Build history of the part. All positions in model axes, mm. A direction names the side the tool comes from. Give positions to 0.01 mm unless a question says otherwise; leave off trailing zeros. Order: outer loops, then holes, each group sorted by start corner. A loop starts at its lowest first (then second) coordinate and runs counter-clockwise, first axis right, second up. Notation, with made-up numbers: (-11.75, 46) - (45.25, 46) arc R31 ccw to (45.25, 75) - close; hole circle Ø4 at (27, 68.25). An arc over 180 degrees is marked (long way). Use a Markdown table: item, result. Add a question column.
(1) Which spindle directions (+Z, -Z, +X, -X, +Y, -Y) get a long thin tool onto all of the face, cutting with end or side? Do faces 1 (the face through (-19, 78, 4)), 2 (the face through (-1, 21, 6)), 3 (the face through (0, 6, 3)). Say none if no direction does.
(2) Slice it at C-C (x = -13). Write the cut outline in (y, z).
(3) Slice it at A-A (y = 38). Write the cut outline in (x, z), then the cut area to 3 significant figures.
(4) Slice it at B-B (x = -1.5). Write the cut outline in (y, z), then the cut area to 3 significant figures.
(5) Flat gauge pins, fed straight in: pin 1 (1.5 mm diameter, centred on y = 57, z = 1, fed in from +X); pin 2 (1.5 mm diameter, centred on y = 104, z = 5.5, fed in from +X); pin 3 (7.5 mm diameter, centred on x = 9.5, y = 64, fed in from +Z). Where does each tip first touch, or does it go through?
(6) Wall check: line 1 (Y direction, x = 12, z = 6.5); line 2 (X direction, y = 12, z = 1); line 3 (Y direction, x = -1.5, z = 0.5). Give the ranges that are in metal, low to high.
Autodesk Inventor part; units mm, degrees
ref_plane "SunkenDetailsPlane" through (0, 0, 9) normal (0, 0, 1) x (1, 0, 0)
ref_plane "HolesPlane" through (-11, 95.6898, 6.5) normal (0, 0, 1) x (1, 0, 0)
ref_plane "YZ Plane" through (0, 0, 0) normal (1, 0, 0) x (0, 1, 0)
sketch "Base" plane through (0, 0, 0) normal (0, 0, 1) x (1, 0, 0)
  line L0 (0, -40.5971) -> (0, 168.3327) construction
  arc A0 (-10.75, 0) -> (10.75, 0) centre (0, 0) ccw
  line L1 (10.75, 48) -> (10.75, 0)
  line L2 (-10.75, 0) -> (-10.75, 50)
  line L3 (-19, 62.5716) -> (-16.2211, 52.5512)
  line L4 (-10.75, 50) -> (-16.2211, 52.5512)
  line L5 (-19, 62.5716) -> (-19, 93.5716)
  line L6 (-19, 93.5716) -> (-11.2142, 103.5369)
  line L7 (10.75, 48) -> (46.4584, 93.7046)
  line L8 (46.4584, 93.7046) -> (52.0821, 118.0639)
  arc A1 (52.0821, 118.0639) -> (48.6133, 127.8595) centre (42.6597, 120.2392) ccw
  arc A2 (48.6133, 127.8595) -> (35.0394, 126.1928) centre (42.6597, 120.2392) ccw
  line L9 (34.8364, 125.933) -> (20.2582, 137.3228)
  line L10 (35.0394, 126.1928) -> (34.8364, 125.933)
  arc A3 (20.2582, 137.3228) -> (14.6435, 136.6334) centre (17.7956, 134.1707) ccw
  line L11 (14.6435, 136.6334) -> (-11.2142, 103.5369)
  line L12 (42.6597, 120.2392) -> (48.6133, 127.8595) construction
  dimension "d0" = 142
  dimension "d1" = 155
  dimension "d2" = 21.5
  dimension "d3" = 115
  dimension "d4" = 130.5
  dimension "d7" = 51.5
  dimension "d8" = 18.5
  dimension "d9" = 4
  dimension "d10" = 58
  dimension "d11" = 25
  dimension "d14" = 42
  dimension "d15" = 50
  dimension "d18" = 10
  dimension "d57" = 48
  dimension "d100" = 19
  dimension "d101" = 31
extrude "BaseFeature" add sketch "Base" along normal blind 9
ref_plane "SunkenDetailsPlane" through (0, 0, 9) normal (0, 0, 1) x (1, 0, 0)
sketch "SunkenDetails" plane through (0, 0, 9) normal (0, 0, 1) x (1, 0, 0)
  line L0 (0.9151, 89.8249) -> (26.6729, 122.7934)
  line L1 (4.8551, 86.7466) -> (30.613, 119.7151)
  arc A0 (30.613, 119.7151) -> (26.6729, 122.7934) centre (28.6429, 121.2543) ccw
  line L2 (0.9151, 97.9462) -> (24.272, 127.8418)
  line L3 (24.272, 127.8418) -> (20.332, 130.9201)
  line L4 (16.1209, 130.403) -> (0.9151, 110.9404)
  arc A1 (20.332, 130.9201) -> (16.1209, 130.403) centre (18.485, 128.556) ccw
  line L5 (-4, 91.6552) -> (-4, 104.6494)
  line L6 (-4, 104.6494) -> (-11, 95.6898)
  line L7 (-11, 95.6898) -> (-11, 55.6335)
  line L8 (-11, 55.6335) -> (-4, 52.3693)
  line L9 (-4, 77.8836) -> (-4, 52.3693)
  arc A2 (-6.1033, 88.9631) -> (-4, 77.8836) centre (-0.1932, 84.3457) ccw
  line L10 (-6.1033, 88.9631) -> (-4, 91.6552)
  line L11 (5.75, 42.3059) -> (5.75, 0)
  line L12 (-5.75, 47.6685) -> (5.75, 42.3059)
  line L13 (-5.75, 0) -> (-5.75, 47.6685)
  arc A3 (-5.75, 0) -> (5.75, 0) centre (0, 0) ccw
  line L14 (4.6626, 48.3299) -> (26.8264, 76.6983)
  line L15 (3.3496, 76.6983) -> (26.8264, 76.6983)
  line L16 (1, 73.6909) -> (3.3496, 76.6983)
  arc A4 (0.9151, 89.8249) -> (4.8551, 86.7466) centre (2.8851, 88.2857) ccw
  line L17 (7.256, 81.6983) -> (30.7329, 81.6983)
  line L18 (7.256, 81.6983) -> (39.1705, 122.5469)
  line L19 (30.7329, 81.6983) -> (41.8359, 95.9094)
  line L20 (41.8359, 95.9094) -> (47.1112, 118.7594)
  arc A5 (47.1112, 118.7594) -> (39.1705, 122.5469) centre (42.721, 119.7729) ccw
  line L21 (10.75, 0) -> (10.75, 48) construction
  arc A6 (-10.75, 0) -> (10.75, 0) centre (0, 0) ccw construction
  line L22 (10.75, 0) -> (10.75, 48) construction
  line L23 (10.75, 48) -> (46.4584, 93.7046) construction
  line L24 (46.4584, 93.7046) -> (52.0821, 118.0639) construction
  arc A7 (52.0821, 118.0639) -> (35.0394, 126.1928) centre (42.6597, 120.2392) ccw construction
  line L25 (35.0394, 126.1928) -> (34.8364, 125.933) construction
  line L26 (34.8364, 125.933) -> (20.2582, 137.3228) construction
  arc A8 (20.2582, 137.3228) -> (14.6435, 136.6334) centre (17.7956, 134.1707) ccw construction
  line L27 (14.6435, 136.6334) -> (-19, 93.5716) construction
  line L28 (-19, 93.5716) -> (-19, 62.5716) construction
  line L29 (-19, 62.5716) -> (-16.2211, 52.5512) construction
  line L30 (-16.2211, 52.5512) -> (-10.75, 50) construction
  line L31 (-10.75, 50) -> (-10.75, 0) construction
  line L32 (-10.75, 50) -> (-10.75, 0) construction
  line L33 (10.75, 48) -> (46.4584, 93.7046) construction
  line L34 (-19, 93.5716) -> (-19, 62.5716) construction
  line L35 (14.6435, 136.6334) -> (-19, 93.5716) construction
  line L36 (46.4584, 93.7046) -> (52.0821, 118.0639) construction
  line L37 (34.8364, 125.933) -> (20.2582, 137.3228) construction
  arc A9 (-10.75, 0) -> (10.75, 0) centre (0, 0) ccw construction
  line L38 (24.272, 127.8418) -> (30.1821, 123.2243) construction
  line L39 (-10.75, 50) -> (-5.75, 47.6685) construction
  line L40 (-16.2211, 52.5512) -> (-10.75, 50) construction
  line L41 (2.8851, 88.2857) -> (-0.1932, 84.3457) construction
  line L42 (0.9151, 110.9404) -> (0.9151, 97.9462)
  line L43 (0.9151, 97.9462) -> (-4, 91.6552) construction
  line L44 (0.9151, 97.9462) -> (0.9151, 89.8249) construction
  line L45 (39.1705, 122.5469) -> (34.8364, 125.933) construction
  line L46 (1.346, 86.3157) -> (7.256, 81.6983) construction
  line L47 (1, 73.6909) -> (1, 50.0378)
  line L48 (1, 50.0378) -> (4.6626, 48.3299)
  point P0 (-11.2142, 103.5369)
  dimension "d23" = 5
  dimension "d30" = 8
  dimension "d32" = 5
  dimension "d34" = 5
  dimension "d35" = 5
  dimension "d36" = 5
  dimension "d49" = 5
  dimension "d54" = 5
  dimension "d59" = 5
  dimension "d60" = 5
  dimension "d61" = 5
  dimension "d66" = 5
  dimension "d76" = 3
  dimension "d77" = 7
  dimension "d102" = 5
  dimension "d103" = 5
  dimension "d104" = 36
extrude "SunkenDetailsFeature" cut sketch "SunkenDetails" against normal blind 5 contours L0 A0 L1 A4 | L42 L4 A1 L3 L2 | L10 A2 L9 L8 L7 L6 L5 | L48 L47 L16 L15 L14 | L18 A5 L20 L19 L17
ref_plane "HolesPlane" through (-11, 95.6898, 6.5) normal (0, 0, 1) x (1, 0, 0)
sketch "Holes" plane through (-11, 95.6898, 6.5) normal (0, 0, 1) x (1, 0, 0)
  circle A0 centre (21.6537, 21.2184) radius 3
  circle A1 centre (28.426, 29.8865) radius 3
  circle A2 centre (11, -57.6898) radius 3
  circle A3 centre (11, -68.6898) radius 3
  line L0 (8, -77.6898) -> (8, -86.6898)
  arc A4 (8, -86.6898) -> (14, -86.6898) centre (11, -86.6898) ccw
  line L1 (14, -86.6898) -> (14, -77.6898)
  arc A5 (14, -77.6898) -> (8, -77.6898) centre (11, -77.6898) ccw
  circle A6 centre (11, -95.6898) radius 3
  line L2 (11.9151, 15.2506) -> (27.1209, 34.7132) construction
  line L3 (35.272, 32.152) -> (11.9151, 2.2564) construction
  line L4 (21.6537, 21.2184) -> (28.426, 29.8865) construction
  line L5 (31.332, 35.2303) -> (35.272, 32.152)
  arc A7 (0.25, -95.6898) -> (21.75, -95.6898) centre (11, -95.6898) ccw construction
  line L6 (0.25, -45.6898) -> (0.25, -95.6898) construction
  line L7 (21.75, -95.6898) -> (21.75, -47.6898) construction
  line L8 (11, -57.6898) -> (11, -95.6898) construction
  dimension "d83" = 6
  dimension "d84" = 9
  dimension "d85" = 9
  dimension "d86" = 9
  dimension "d87" = 11
  dimension "d88" = 8
  dimension "d89" = 11
  dimension "d90" = 4
  dimension "d91" = 6
extrude "HolesFeature" cut sketch "Holes" against normal through all
extrude "SunkenDetailFeature" cut sketch "SunkenDetails" against normal blind 3 contours L11 A3 L13 L12
chamfer "DetailChamfersFeature" distance 1 angle 45 9 edges at (0.9151, 97.9462, 6.5) (-4, 104.6494, 6.5) (-11, 95.6898, 6.5) (-5.75, 47.6685, 7.5) (5.75, 42.3059, 7.5) (-4, 52.3693, 6.5) (7.256, 81.6983, 6.5) (4.6626, 48.3299, 6.5) (-11, 55.6335, 6.5)
sketch "Logo" plane through (0, 0, 4) normal (0, 0, 1) x (1, 0, 0)
  line L0 (6, 71.6983) -> (7.5, 71.6983)
  line L1 (7.5, 71.6983) -> (7.5, 68.1983)
  line L2 (9.5, 73.6983) -> (4, 73.6983)
  line L3 (9.5, 66.1983) -> (9.5, 73.6983)
  line L4 (11.5, 66.1983) -> (11.5, 73.6983)
  line L5 (14.5, 65.1983) -> (4, 65.1983)
  line L6 (14.5, 74.6983) -> (14.5, 65.1983)
  line L7 (13.5, 66.1983) -> (11.5, 66.1983)
  line L8 (13.5, 73.6983) -> (13.5, 66.1983)
  line L9 (3, 74.6983) -> (14.5, 74.6983)
  line L10 (11.5, 73.6983) -> (13.5, 73.6983)
  line L11 (6, 68.1983) -> (6, 71.6983)
  line L12 (4, 73.6983) -> (4, 66.1983)
  line L13 (3, 66.1983) -> (3, 74.6983)
  line L14 (4, 66.1983) -> (9.5, 66.1983)
  line L15 (4, 66.1983) -> (4, 65.1983)
  line L16 (3, 66.1983) -> (4, 66.1983)
  line L17 (7.5, 68.1983) -> (6, 68.1983)
  line L18 (3.3496, 76.6983) -> (26.8264, 76.6983) construction
  line L19 (1, 50.0378) -> (1, 73.6909) construction
  dimension "d140" = 1
  dimension "d141" = 1
  dimension "d142" = 1
  dimension "d143" = 1
  dimension "d144" = 2
  dimension "d145" = 1.5
  dimension "d146" = 2
  dimension "d147" = 2
  dimension "d148" = 2
  dimension "d149" = 9.5
  dimension "d150" = 2
  dimension "d151" = 2
  dimension "d152" = 2
  dimension "d153" = 2
extrude "LogoFeature" cut sketch "Logo" against normal blind 1
properties part number "ShinConnector"
Solution:
| question | item | result |
|---|---|---|
| 1 | face 1 | +Z, -Z, -X, +Y, -Y |
| 1 | face 2 | +Z |
| 1 | face 3 | +Z, -Z |
| 2 | outline | (51.05, 0) - (101.25, 0) - (101.25, 9) - (51.05, 9) - close |
| 3 | outline | (-10.75, 0) - (-3, 0) - (-3, 6) - (-5.75, 6) - (-5.75, 9) - (-10.75, 9) - close; (3, 0) - (10.75, 0) - (10.75, 9) - (5.75, 9) - (5.75, 6) - (3, 6) - close |
| 3 | area | 123 mm2 |
| 4 | outline | (-10.64, 0) - (-2.6, 0) - (-2.6, 6) - (-5.55, 6) - (-5.55, 9) - (-10.64, 9) - close; (2.6, 0) - (6.4, 0) - (6.4, 6) - (2.6, 6) - close; (20.6, 0) - (24.4, 0) - (24.4, 6) - (20.6, 6) - close; (29.6, 0) - (35.4, 0) - (35.4, 6) - (29.6, 6) - close; (40.6, 0) - (115.97, 0) - (115.97, 9) - (45.69, 9) - (45.69, 6) - (40.6, 6) - close |
| 4 | area | 807 mm2 |
| 5 | pin 1 | x = 18.37 |
| 5 | pin 2 | x = 49.01 |
| 5 | pin 3 | z = 4 |
| 6 | line 1 | 49.6 to 57.72, 76.7 to 81.7, 87.77 to 95.89, 104.01 to 112.13, 125.13 to 133.25 |
| 6 | line 2 | -10.75 to -3, 3 to 10.75 |
| 6 | line 3 | -10.64 to -2.6, 2.6 to 6.4, 20.6 to 24.4, 29.6 to 35.4, 40.6 to 115.97 |
